Autodesk Inventor part; units mm, degrees
ref_plane "YZ Plane" through (0, 0, 0) normal (1, 0, 0) x (0, 1, 0)
ref_plane "XZ Plane" through (0, 0, 0) normal (0, 1, 0) x (-1, 0, 0)
ref_plane "XY Plane" through (0, 0, 0) normal (0, 0, 1) x (1, 0, 0)
sketch "Esboço1" plane through (0, 0, 0) normal (0, 1, 0) x (-1, 0, 0)
  arc A0 (-0.2821, 5) -> (-1.282, 4) centre (-0.282, 4) ccw
  line L0 (-1.282, 4) -> (-1.282, 0.6875)
  arc A1 (-2.282, -0.3125) -> (-1.282, 0.6875) centre (-2.282, 0.6875) ccw
  line L1 (-2.282, -0.3125) -> (-5, -0.3125)
  arc A2 (-5, -0.3125) -> (-6, -1.3125) centre (-5, -1.3125) ccw
  line L2 (-6, -1.3125) -> (-6, -4)
  arc A3 (-6, -4) -> (-5, -5) centre (-5, -4) ccw
  line L3 (-5, -5) -> (5, -5)
  arc A4 (5, -5) -> (6, -4) centre (5, -4) ccw
  line L4 (6, -4) -> (6, 4)
  arc A5 (6, 4) -> (5, 5) centre (5, 4) ccw
  line L5 (5, 5) -> (-0.2821, 5)
  circle A6 centre (3.0146, -1.9633) radius 0.45
  circle A7 centre (-3.8014, -2.7994) radius 1.25
  circle A8 centre (3.8014, 2.7994) radius 1.25
  circle A9 centre (3.8014, 2.7994) radius 1.25
  circle A10 centre (3.8014, 2.7994) radius 0.75
  circle A11 centre (-3.8014, -2.7994) radius 1.25
  circle A12 centre (-3.8014, -2.7994) radius 0.75
  circle A13 centre (0, 0) radius 0.5
  circle A14 centre (0, 3) radius 0.45
  dimension "d9" = 1
  dimension "d12" = 0.9
  dimension "d13" = 2
extrude "Extrusão1" add sketch "Esboço1" along normal blind 0.8 contours L5 A5 L4 A4 L3 A3 L2 A2 L1 A1 L0 A0 | A14
extrude "Extrusão2" add sketch "Esboço1" along normal blind 0.4 contours A7 | A8
sketch "Esboço2" plane through (0, 0, 0) normal (0, -1, 0) x (1, 0, 0)
  circle A0 centre (-3.8014, 2.7994) radius 0.75
  circle A1 centre (-3.8014, 2.7994) radius 1.5
  circle A2 centre (3.8014, -2.7994) radius 0.75
  circle A3 centre (3.8014, -2.7994) radius 1.5
  point P0 (0, 0)
  dimension "d4" = 3
  dimension "d5" = 3
extrude "Extrusão3" add sketch "Esboço2" along normal blind 2.8
extrude "Extrusão4" cut sketch "Esboço1" along normal blind 10 contours A14
properties part number "Chapa Intermediária"
Design review of the part built by this model. Coordinates are the model's own, in mm. A direction names the side the tool comes from. Give positions to 0.01 mm unless a question says otherwise; leave off trailing zeros. Loops run counter-clockwise (first coordinate to the right, second up) from the corner with the lowest first, then second, coordinate; pieces in that order, holes last. Notation, with made-up numbers: M 20,62 L 60,62 A14 ccw 60,79 Z; hole C -31.5,-15 d6. An arc over 180 degrees is marked long. Write item = value, one per line.
Q1. To check wall thickness, follow line 1 (Z direction, x = 0, y = 0.4); line 2 (X direction, y = -1.5, z = 2.75); line 3 (Y direction, x = -2, z = 0.25). State the ranges of each line that lie inside material, in increasing order. Write a range as [from, to].
Output values:
line_1 = [-5, -0.5], [0.5, 2.55], [3.45, 5]
line_2 = [-5.3, -4.55], [-3.05, -2.3]
line_3 = [0, 0.8]
Q2. We need section C-C (x = -4.25). Give the boundary of the cut face in (y, z), plus the area to 3 significant figures.
Output values:
outline = M -2.8,1.37 L 0,1.37 L 0,-5 L 0.8,-5 L 0.8,1.63 L 0.4,1.63 L 0.4,2.2 L -2.8,2.2 Z; M -2.8,3.4 L 0.4,3.4 L 0.4,3.97 L 0.8,3.97 L 0.8,5 L 0,5 L 0,4.23 L -2.8,4.23 Z
area = 11.2 mm^2
Q3. Insertion check: pin 1 (1.5 mm diameter, centred on y = 0, z = 4, fed in from +X); pin 2 (5 mm diameter, centred on x = -0.5, z = -2, fed in from -Y); pin 3 (1.2 mm diameter, centred on x = -3.8, z = 2.8, fed in from -Y); pin 4 (2 mm diameter, centred on x = 3.8, z = -2.8, fed in from +Y). Each pin has a flat end and moves straight along its axis. Give the tip position at first contact, or say it passes through.
Output values:
pin_1 = 1.28
pin_2 = 0
pin_3 = through
pin_4 = 0.4
Q4. Draft analysis for pull direction Z (two halves, no side actions). For faces 4 (the cylindrical face through (-4.994, 0.597, 2.424)), 5 (the cylindrical face through (1.567, 0.394, -0.012)), 6 (the flat face through (-3, -2.8, 2)), state which applies: +Z half, -Z half, draft (parallel to the pull), parting line (faces both ways), or undercut.
Output values:
face_4 = undercut
face_5 = +Z half
face_6 = draft
Q5. For faces 1 (the cylindrical face through (4.07, 0.6, -1.58)), 2 (the cylindrical face through (-2.416, -1.38, 3.374)), 3 (the cylindrical face through (0.997, 0.394, 4.699)), list the 3-axis set-ups (+Z, -Z, +X, -X, +Y, -Y) from which the entire face can be reached by the end or side of a thin tool; tool diameter is ignored.
Output values:
face_1 = +Y
face_2 = -Y
face_3 = +Z, +X, +Y, -Y
Q6. We need section B-B (z = 3). Give the boundary of the cut face in (x, y), plus the area to 3 significant figures.
Output values:
outline = M -6,0 L -5.29,0 L -5.29,-2.8 L -4.52,-2.8 L -4.52,0.4 L -5.04,0.4 L -5.04,0.8 L -6,0.8 Z; M -3.08,-2.8 L -2.31,-2.8 L -2.31,0 L -0.45,0 L -0.45,0.8 L -2.57,0.8 L -2.57,0.4 L -3.08,0.4 Z; M 0.45,0 L 1.28,0 L 1.28,0.8 L 0.45,0.8 Z
area = 7.82 mm^2
Q7. We need section A-A (x = 0). Give the boundary of the cut face in (y, z).
Output values:
outline = M 0,-5 L 0.8,-5 L 0.8,-0.5 L 0,-0.5 Z; M 0,0.5 L 0.8,0.5 L 0.8,2.55 L 0,2.55 Z; M 0,3.45 L 0.8,3.45 L 0.8,5 L 0,5 Z
Q8. We need section D-D (z = 0.25). Give the boundary of the cut face in (x, y).
Output values:
outline = M -6,0 L -0.43,0 L -0.43,0.8 L -6,0.8 Z; M 0.43,0 L 1.38,0 L 1.38,0.8 L 0.43,0.8 Z
